Verification items for this drawing (mm, ordinates from the low corner). Round coordinates to 2 decimals unless told otherwise and drop trailing zeros. Order: outer loops, then holes, each group sorted by start corner. A loop starts at its lowest first (then second) coordinate and runs counter-clockwise, first axis right, second up. Notation, with made-up numbers: (42, 46.25) -> (97, 46.25) arc R16 ccw to (97, 59.25) -> close; hole circle Ø10 at (67, -2.75). An arc over 180 degrees is marked (long way). Answer in a Markdown table with one row per item.
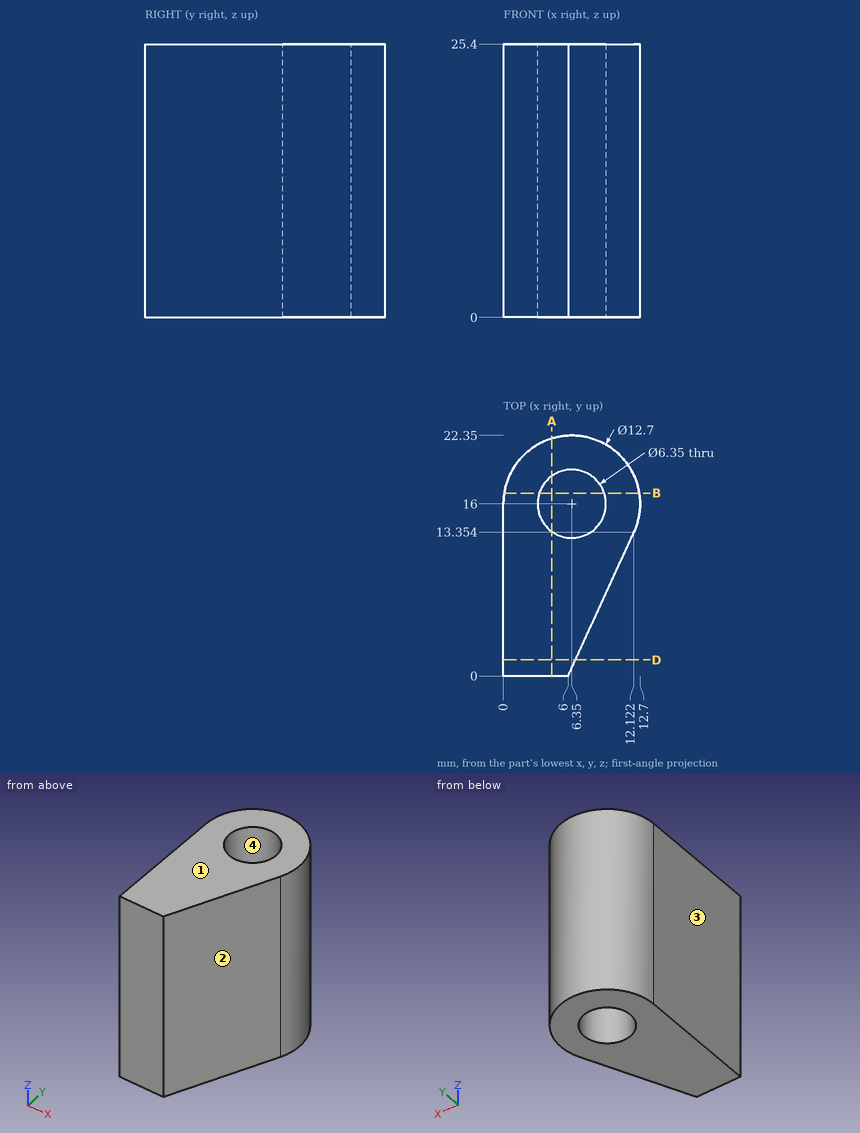
Item 1: Scan lines: line 1 (X direction, y = 17.25, z = 9.75) (1 decimal); line 2 (X direction, y = 16.5, z = 8.75) (1 decimal); line 3 (X direction, y = 5, z = 13). Record each from-to range of solid material in increasing order. Write a range as [from, to].
Result sheet:
| item | result |
|---|---|
| line 1 | x = [0.1, 3.4], [9.3, 12.6] |
| line 2 | x = [0, 3.2], [9.5, 12.7] |
| line 3 | x = [0, 8.29] |
Item 2: Cross-section at D-D (y = 1.5). Record the boundary of the cut face in (x, z).
Result sheet:
| item | result |
|---|---|
| outline | (0, 0) -> (6.69, 0) -> (6.69, 25.4) -> (0, 25.4) -> close |
Item 3: Cross-section at A-A (x = 4.5). Record the boundary of the cut face in (y, z) (1 decimal).
Result sheet:
| item | result |
|---|---|
| outline | (0, 0) -> (13.4, 0) -> (13.4, 25.4) -> (0, 25.4) -> close; (18.6, 0) -> (22.1, 0) -> (22.1, 25.4) -> (18.6, 25.4) -> close |
Item 4: Cross-section at B-B (y = 17). Record the boundary of the cut face in (x, z).
Result sheet:
| item | result |
|---|---|
| outline | (0.08, 0) -> (3.34, 0) -> (3.34, 25.4) -> (0.08, 25.4) -> close; (9.36, 0) -> (12.62, 0) -> (12.62, 25.4) -> (9.36, 25.4) -> close |
Item 5: Mould release check, pull along X, two halves, no side actions. Record for the marked faces 1, 2, 3 and 4: pulls with the +X half, pulls with the -X half, needs draft (parallel to the pull), parting line crosses it, or undercut.
Result sheet:
| item | result |
|---|---|
| face 1 | needs draft |
| face 2 | pulls with the +X half |
| face 3 | pulls with the -X half |
| face 4 | undercut |
Item 6: Depth check by flat-ended pin: P1, Ø3, axis at x = 7, y = 16.5, coming from the +Z side; P2, Ø1, axis at x = 1.5, z = 22.5, coming from the +Y side (1 decimal). Enter the tip coordinate at first touch or a pass-through.
Result sheet:
| item | result |
|---|---|
| P1 | passes through |
| P2 | stops at y = 20.6 |
